Verification items for the finished model (mm, model axes). A direction names the side the tool comes from. Coordinates: 2 decimals unless noted, no trailing zeros. Loops run counter-clockwise (first coordinate to the right, second up) from the corner with the lowest first, then second, coordinate; pieces in that order, holes last. Notation, with made-up numbers: (81, -24) - (112, -24) arc R25 cw to (112, -9) - close; hole circle Ø4 at (52, -2.5). An arc over 180 degrees is marked (long way). One line per item, written item: value. Start each with the question number.
(1) Draft check along Y on faces 1 (the face through (-3, 0, 2)), 2 (the face through (1.3, -1.3, 0)), 3 (the face through (0, 0, 0.7)). Enter one of: +Y half, -Y half, draft (parallel to the pull), parting line (faces both ways), or undercut.
(2) Section check B-B (z = -6.25). Record the boundary of the cut face in (x, y).
(3) Section check C-C (y = 0.65). Record the boundary of the cut face in (x, z), plus the area to 3 significant figures.
(4) Section check D-D (x = 2.55). Record the boundary of the cut face in (y, z).
(5) Gauge pin test, flat ends, axial feed: P1, Ø2, axis at x = -0.5, z = -3.5, coming from the -Y side; P2, Ø3, axis at y = 2, z = -2, coming from the -X side. Record the tip position at first contact, or that the pin passes through.
(6) Thickness scan on probe 1 along X at (y, z) = (0.1, -12.5); probe 2 along Z at (x, y) = (-2.7, 1); probe 3 along Z at (x, y) = (-0.1, 1.25). Record the ranges inside material, lowest first. Write a range as [from, to].
(7) Set-up check for faces 4 (the face through (0, -1.75, 2)), 5 (the face through (-1.5, 0.07, -7.4)), 6 (the face through (0, 0, -15)): record each of +Z, -Z, +X, -X, +Y, -Y from which the full face is reachable in a straight line by a thin tool's end or side.
(8) Section check A-A (x = 0). Record the boundary of the cut face in (y, z), plus the area to 3 significant figures.
```python
from build123d import *

# Parameters (mm, degrees)
SKETCH1_R                   = 3
HEAD_BOSS_EXTRUDE1_DEPTH    = 3.5
HEAD_HEX_CUT_EXTRUDE1_DEPTH = 2.8
SKETCH2_R                   = 1.5
SCREW_BOSS_EXTRUDE2_DEPTH   = 15


with BuildPart() as part:
    # Sketch1 → Head Boss-Extrude1 (new body)
    with BuildSketch(Plane.XY):
        Circle(SKETCH1_R)
    extrude(amount=HEAD_BOSS_EXTRUDE1_DEPTH)

    # Sketch3 → Head Hex Cut-Extrude1 (cut)
    with BuildSketch(Plane.XY.offset(3.5)):
        Polygon((-1.010362971, 1.75), (1.010362971, 1.75), (2.020725942, 0), (1.010362971, -1.75), (-1.010362971, -1.75), (-2.020725942, 0), align=None)
    extrude(amount=-HEAD_HEX_CUT_EXTRUDE1_DEPTH, mode=Mode.SUBTRACT)

    # Sketch2 → Screw Boss-Extrude2 (add)
    with BuildSketch(Plane.XY):
        Circle(SKETCH2_R)
    extrude(amount=-SCREW_BOSS_EXTRUDE2_DEPTH)


solid = part.part
```
Responses:
1. face 1: parting line
1. face 2: draft
1. face 3: undercut
2. outline: circle Ø3 at (0, 0)
3. outline: (-2.93, 0) - (-1.35, 0) - (-1.35, -15) - (1.35, -15) - (1.35, 0) - (2.93, 0) - (2.93, 3.5) - (1.65, 3.5) - (1.65, 0.7) - (-1.65, 0.7) - (-1.65, 3.5) - (-2.93, 3.5) - close
3. area: 51.8 mm²
4. outline: (-1.58, 0) - (1.58, 0) - (1.58, 3.5) - (-1.58, 3.5) - close
5. P1: stops at y = -1.5
5. P2: stops at x = -1.41
6. probe 1: x = [-1.5, 1.5]
6. probe 2: z = [0, 3.5]
6. probe 3: z = [-15, 0.7]
7. face 4: +Z
7. face 5: -Z
7. face 6: -Z, +X, -X, +Y, -Y
8. outline: (-3, 0) - (-1.5, 0) - (-1.5, -15) - (1.5, -15) - (1.5, 0) - (3, 0) - (3, 3.5) - (1.75, 3.5) - (1.75, 0.7) - (-1.75, 0.7) - (-1.75, 3.5) - (-3, 3.5) - close
8. area: 56.2 mm²
